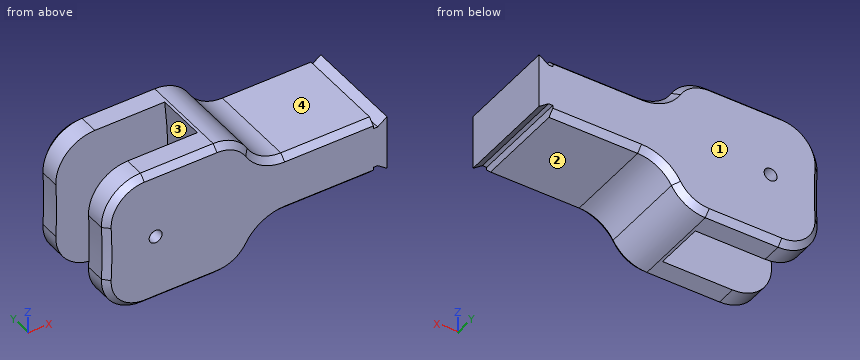
from build123d import *

# Parameters (mm, degrees)
SKETCH2_OUTSIDE_W     = 472.576
SKETCH2_OUTSIDE_H     = 472.576
SKETCH2_OUTSIDE_W_2   = 39.636477918
SKETCH2_OUTSIDE_H_2   = 35
CUT_EXTRUDE1_DEPTH    = 377.781288533
BOSS_EXTRUDE1_DEPTH   = 25.7
BOSS_EXTRUDE2_DEPTH   = 25.7
FILLET1_R             = 10
M4X0_7_TAPPED_HOLE1_D = 3.3
FILLET2_R             = 10
CHAMFER1_SIZE         = 1.5


with BuildPart() as part:
    # Sketch1 → Revolve1 (revolve)
    with BuildSketch(Plane.XY, mode=Mode.PRIVATE) as revolve1_sk:
        Polygon((0, 0), (28.575, 0), (28.575, 12.7), (0, 12.7), (0, 19.2), (38.575, 19.2), (38.575, -6.5), (0, -6.5), align=None)
    revolve(revolve1_sk.sketch.rotate(Axis((-144.78715491, 19.2, 0), (0, -1, 0)), 90), axis=Axis((-144.78715491, 19.2, 0), (0, -1, 0)))

    # Sketch2 outside → Cut-Extrude1 (cut, through all)
    with BuildSketch(Plane(origin=(0, 19.2, 0), x_dir=(1, 0, 0), z_dir=(0, 1, 0))):
        with Locations((-144.787, 0)):
            Rectangle(SKETCH2_OUTSIDE_W, SKETCH2_OUTSIDE_H)
        with Locations((18.756761041, 0)):
            Rectangle(SKETCH2_OUTSIDE_W_2, SKETCH2_OUTSIDE_H_2, mode=Mode.SUBTRACT)
    extrude(amount=-CUT_EXTRUDE1_DEPTH, mode=Mode.SUBTRACT)

    # Sketch3 → Boss-Extrude1 (add, through all)
    with BuildSketch(Plane(origin=(0, 19.2, 0), x_dir=(1, 0, 0), z_dir=(0, 1, 0))):
        with BuildLine():
            Line((38.421550814, 7.5), (68.421550814, 7.5))
            Line((68.421550814, 7.5), (68.421550814, -7.5))
            Line((68.421550814, -7.5), (38.421550814, -7.5))
            ThreePointArc((38.421550814, -7.5), (38.575, 0), (38.421550814, 7.5))
        make_face()
    extrude(amount=-BOSS_EXTRUDE1_DEPTH)

    # Sketch4 → Boss-Extrude2 (add, through all)
    with BuildSketch(Plane(origin=(0, 19.2, 0), x_dir=(1, 0, 0), z_dir=(0, 1, 0))):
        Polygon((71.921550814, 7), (71.921550814, -7), (69.511550814, -5.25), (68.421550814, -5.25), (68.421550814, 5.25), (69.511550814, 5.25), align=None)
    extrude(amount=-BOSS_EXTRUDE2_DEPTH)

    # Fillet1
    fillet1_edges = [part.edges().sort_by_distance(p)[0] for p in [
        (-1.061477918, 15.95, 17.5),
        (-1.061477918, -3.25, 17.5),
        (-1.061477918, -3.25, -17.5),
        (-1.061477918, 15.95, -17.5),
        (37.73799364, 6.35, -17.5),
        (37.73799364, 6.35, 17.5),
    ]]
    fillet(fillet1_edges, radius=FILLET1_R)

    # M4x0.7 Tapped Hole1 (through all)
    with Locations(Plane(origin=(0, 19.2, 0), x_dir=(1, 0, 0), z_dir=(0, 1, 0))):
        with Locations((12.7, 0)):
            Hole(M4X0_7_TAPPED_HOLE1_D / 2)

    # Fillet2
    fillet2_edges = [part.edges().sort_by_distance(p)[0] for p in [
        (38.421550814, 6.35, 7.5),
        (38.421550814, 6.35, -7.5),
    ]]
    fillet(fillet2_edges, radius=FILLET2_R)

    # Chamfer1
    chamfer1_edges = [part.edges().sort_by_distance(p)[0] for p in [
        (19.115441742, 19.2, 17.5),
        (2.577841169, 19.2, 14.397631358),
        (2.577841169, 19.2, -14.397631358),
        (33.41269138, 19.2, 16.160254038),
        (33.41269138, -6.5, 16.160254038),
        (57.077375135, 19.2, 7.5),
        (57.077375135, -6.5, 7.5),
        (33.41269138, 19.2, -16.160254038),
        (40.733199456, 19.2, 8.839745962),
        (40.733199456, -6.5, 8.839745962),
        (40.733199456, 19.2, -8.839745962),
        (40.733199456, -6.5, -8.839745962),
        (57.077375135, -6.5, -7.5),
        (57.077375135, 19.2, -7.5),
        (19.115441742, 19.2, -17.5),
        (19.115441742, -6.5, -17.5),
        (19.115441742, -6.5, 17.5),
        (0, -6.5, 0),
        (2.577841169, -6.5, 14.397631358),
        (2.577841169, -6.5, -14.397631358),
        (33.41269138, -6.5, -16.160254038),
        (0, 19.2, 0),
    ]]
    chamfer(chamfer1_edges, length=CHAMFER1_SIZE)


solid = part.part
Here's how the part is built. I have some questions about the finished solid (model axes, mm). Face numbers are marked on the shaded views. Round coordinates to 2 decimals unless told otherwise and drop trailing zeros. Write each loop counter-clockwise with the first axis right and the second up, starting at its lowest first coordinate (ties: lowest second). Pieces come first, ordered by that corner, then holes.
1. If we mould it in two halves opening along Z, with no side actions, what happens to the marked faces 1, 2, 3 and 4? For each: released by +Z, released by -Z, zero draft, split by the parting line, or undercut.
2. Suppose I cut it at C-C (x = 24). List the corners of the cut face in (y, z) for me, and give its area (4 significant figures).
3. Suppose I cut it at A-A (x = 12.7). List the corners of the cut face in (y, z) for me, and give its area (3 significant figures).
4. I need wall thicknesses on L1, parallel to Y at x = 17.5, z = -2; L2, parallel to Z at x = 12.7, y = 17.5; L3, parallel to Z at x = 14, y = -3.25. Which ranges of each line are inside material? Lowest first, please.
5. Suppose I cut it at D-D (x = 54.5). List the corners of the cut face in (y, z) for me, and give its area (3 significant figures).
6. Will these pins go through, and if not, where does the flat tip stop? pin 1 Ø8 at (x, y) = (64, 11.5) entering from -Z; pin 2 Ø3 at (x, y) = (32.5, 4.5) entering from -Z; pin 3 Ø0.5 at (x, y) = (69, 5.5) entering from -Z; pin 4 Ø2.5 at (x, z) = (12.7, 0) entering from -Y.
7. Suppose I cut it at B-B (z = 0). List the corners of the cut face in (x, y) for me (3 decimals), and give its area (3 significant figures).
Answer sheet:
1. face 1: zero draft
1. face 2: released by -Z
1. face 3: undercut
1. face 4: released by +Z
2. outline: (-6.5, -16) - (-5, -17.5) - (0, -17.5) - (0, 17.5) - (-5, 17.5) - (-6.5, 16) - close; (12.7, -17.5) - (17.7, -17.5) - (19.2, -16) - (19.2, 16) - (17.7, 17.5) - (12.7, 17.5) - close
2. area: 450.5 mm2
3. outline: (-6.5, -16) - (-5, -17.5) - (0, -17.5) - (0, -1.65) - (-6.5, -1.65) - close; (-6.5, 1.65) - (0, 1.65) - (0, 17.5) - (-5, 17.5) - (-6.5, 16) - close; (12.7, -17.5) - (17.7, -17.5) - (19.2, -16) - (19.2, -1.65) - (12.7, -1.65) - close; (12.7, 1.65) - (19.2, 1.65) - (19.2, 16) - (17.7, 17.5) - (12.7, 17.5) - close
3. area: 408 mm2
4. L1: y = -6.5 to 0, 12.7 to 19.2
4. L2: z = -17.5 to -1.65, 1.65 to 17.5
4. L3: z = -17.5 to -1.02, 1.02 to 17.5
5. outline: (-6.5, -6) - (-5, -7.5) - (17.7, -7.5) - (19.2, -6) - (19.2, 6) - (17.7, 7.5) - (-5, 7.5) - (-6.5, 6) - close
5. area: 381 mm2
6. pin 1: stops at z = -7.5
6. pin 2: stops at z = -17.16
6. pin 3: stops at z = -5.25
6. pin 4: passes through
7. outline: (0, -5) - (1.5, -6.5) - (11.05, -6.5) - (11.05, 0) - (0, 0) - close; (0, 12.7) - (11.05, 12.7) - (11.05, 19.2) - (1.5, 19.2) - (0, 17.7) - close; (14.35, -6.5) - (71.922, -6.5) - (71.922, 19.2) - (14.35, 19.2) - (14.35, 12.7) - (28.575, 12.7) - (28.575, 0) - (14.35, 0) - close
7. area: 1,440 mm2
